Here's how the part is built. I have some questions about the finished solid (model axes, mm). Face numbers are marked on the shaded views. A direction names the side the tool comes from. Round coordinates to 2 decimals unless told otherwise and drop trailing zeros. Write each loop counter-clockwise with the first axis right and the second up, starting at its lowest first coordinate (ties: lowest second). Pieces come first, ordered by that corner, then holes. Notation, with made-up numbers: (67.5, 60.25) - (125.5, 60.25) arc R15 ccw to (125.5, 85.25) - close; hole circle Ø4 at (88.25, 69). An arc over 180 degrees is marked (long way). Write item = value, one per line. Start each with the question number.
Item 1: If we section it at B-B (y = 7): Please give me the cut outline in (x, z), and give its area (3 significant figures).
Item 2: Which directions (+Z, -Z, +X, -X, +Y, -Y) give clear straight access to the entire face, cutting with the end or side of a thin tool? Please do the marked faces 1, 2 and 3.
Item 3: If I drill on line 1 along X through (y, z) = (2, -6.75); line 2 along Z through (x, y) = (39, 7); line 3 along Y through (x, z) = (39.5, 0), over which ranges is the centre line in solid material (lowest first)? Write a range as [from, to].
Item 4: If we section it at C-C (x = 47): Please give me the cut outline in (y, z).
Item 5: For P1, Ø9.5, axis at x = 9.5, z = 10, coming from the +Y side; P2, Ø4, axis at y = 6.5, z = -2.5, coming from the +X side; P3, Ø2, axis at x = 47.5, y = 7.5, coming from the -Z side, each with a flat end and sliding along its axis, tell me the tip position at first contact or that it passes through.
Item 6: If we section it at D-D (z = 0): Please give me the cut outline in (x, y), and give its area (3 significant figures).
Item 7: Thinking about a two-plate mould opening in X: for the marked faces 4, 5, 6 and 7, which applies, pulls with the +X half, pulls with the -X half, needs draft (parallel to the pull), parting line crosses it, or undercut?
Item 8: If we section it at A-A (z = -6.75): Please give me the cut outline in (x, y).
```python
from build123d import *

# Parameters (mm, degrees)
EXTRUDE_2_DEPTH     = 4
SKETCH_7_W          = 100
SKETCH_7_H          = 16
EXTRUDE_3_DEPTH     = 6
SKETCH_8_R          = 5.25
CUT_EXTRUDE_3_DEPTH = 96
SKETCH_9_W          = 30
SKETCH_9_H          = 6
CUT_EXTRUDE_4_DEPTH = 94.680307429
SKETCH_10_R         = 1.8
CUT_EXTRUDE_5_DEPTH = 92.607859925
FILLET_3_R          = 15
CHAMFER_1_SIZE      = 1


with BuildPart() as part:
    # Эскиз6 → Бобышка-Вытянуть2 (new body)
    with BuildSketch(Plane(origin=(0, 0, 0), x_dir=(1, 0, 0), z_dir=(0, 1, 0))):
        Polygon((0, 16), (0, 8), (-10, 8), (-10, -8), (0, -8), (0, -16), (30, -16), (30, -8), (90, -8), (90, 8), (30, 8), (30, 16), align=None)
    extrude(amount=EXTRUDE_2_DEPTH)

    # Эскиз7 → Бобышка-Вытянуть3 (add)
    with BuildSketch(Plane(origin=(0, 4, 0), x_dir=(1, 0, 0), z_dir=(0, 1, 0))):
        with Locations((40, 0)):
            Rectangle(SKETCH_7_W, SKETCH_7_H)
    extrude(amount=EXTRUDE_3_DEPTH)

    # Эскиз8 → Вырез-Вытянуть3 (cut)
    with BuildSketch(Plane(origin=(90, 0, 0), x_dir=(0, 0, -1), z_dir=(1, 0, 0))):
        with Locations((0, 7)):
            Circle(SKETCH_8_R)
    extrude(amount=-CUT_EXTRUDE_3_DEPTH, mode=Mode.SUBTRACT)

    # Эскиз9 → Вырез-Вытянуть4 (cut, through all)
    with BuildSketch(Plane.XY.offset(8)):
        with Locations((15, 7)):
            Rectangle(SKETCH_9_W, SKETCH_9_H)
    extrude(amount=-CUT_EXTRUDE_4_DEPTH, mode=Mode.SUBTRACT)

    # Эскиз10 → Вырез-Вытянуть5 (cut, through all)
    with BuildSketch(Plane(origin=(0, 4, 0), x_dir=(1, 0, 0), z_dir=(0, 1, 0))):
        with Locations(Location((15, -13.5, 0), (0, 0, 270))):
            Circle(SKETCH_10_R)
        with Locations(Location((3.308657049, 6.75, 0), (0, 0, 270))):
            Circle(SKETCH_10_R)
        with Locations(Location((26.691342951, 6.75, 0), (0, 0, 270))):
            Circle(SKETCH_10_R)
    extrude(amount=-CUT_EXTRUDE_5_DEPTH, mode=Mode.SUBTRACT)

    # Скругление3
    # the kernel refuses this fillet: 15 mm, written as the material it takes off along each edge
    with BuildSketch(Plane(origin=(30, -33.166247904, -16), x_dir=(-1, 0, 0), z_dir=(0, 1, 0))) as fillet_3_piece_1:
        with BuildLine():
            CenterArc((13.266499161, 15), FILLET_3_R, 207.818139285, 62.181860715)
            Line((0, 8), (-0.265329983, 7.86))
            ThreePointArc((-0.265329983, 7.86), (-0.3, 4), (-0.3, 0))
            Line((-0.3, 0), (0, -0.3))
            Line((0, -0.3), (13.266499161, -0.3))
            Line((13.266499161, -0.3), (13.266499161, 0))
        make_face()
    extrude(amount=70.332495807, mode=Mode.SUBTRACT)
    with BuildSketch(Plane(origin=(0, -33.166247904, -16), x_dir=(0, 0, 1), z_dir=(0, 1, 0))) as fillet_3_piece_2:
        with BuildLine():
            CenterArc((15, 13.266499161), FILLET_3_R, 180, 62.181860715)
            Line((0, 13.266499161), (-0.3, 13.266499161))
            Line((-0.3, 13.266499161), (-0.3, 0))
            Line((-0.3, 0), (0, -0.3))
            ThreePointArc((0, -0.3), (4, -0.3), (7.86, -0.265329983))
            Line((7.86, -0.265329983), (8, 0))
        make_face()
    extrude(amount=70.332495807, mode=Mode.SUBTRACT)
    with BuildSketch(Plane(origin=(30, -33.166247904, 16), x_dir=(-1, 0, 0), z_dir=(0, 1, 0))) as fillet_3_piece_3:
        with BuildLine():
            CenterArc((13.266499161, -15), FILLET_3_R, 90, 62.181860715)
            Line((0, -8), (-0.265329983, -7.86))
            ThreePointArc((-0.265329983, -7.86), (-0.3, -4), (-0.3, 0))
            Line((-0.3, 0), (0, 0.3))
            Line((0, 0.3), (13.266499161, 0.3))
            Line((13.266499161, 0.3), (13.266499161, 0))
        make_face()
    extrude(amount=70.332495807, mode=Mode.SUBTRACT)
    with BuildSketch(Plane(origin=(0, -33.166247904, 16), x_dir=(0, 0, -1), z_dir=(0, 1, 0))) as fillet_3_piece_4:
        with BuildLine():
            CenterArc((15, -13.266499161), FILLET_3_R, 117.818139285, 62.181860715)
            Line((0, -13.266499161), (-0.3, -13.266499161))
            Line((-0.3, -13.266499161), (-0.3, 0))
            Line((-0.3, 0), (0, 0.3))
            ThreePointArc((0, 0.3), (4, 0.3), (7.86, 0.265329983))
            Line((7.86, 0.265329983), (8, 0))
        make_face()
    extrude(amount=70.332495807, mode=Mode.SUBTRACT)

    # Фаска1
    # the kernel refuses this chamfer: 1 mm, written as the material it takes off along each edge
    with BuildSketch(Plane(origin=(3.308657049, 4, -6.75), x_dir=(0, 0, 1), z_dir=(-1, 0, 0))) as chamfer_1_piece_1:
        Polygon((1.8, -CHAMFER_1_SIZE), (1.8 + CHAMFER_1_SIZE, 0), (1.8, 0), align=None)
    revolve(axis=Axis((3.308657049, 4, -6.75), (0, 1, 0)), mode=Mode.SUBTRACT)
    with BuildSketch(Plane(origin=(26.691342951, 4, -6.75), x_dir=(0, 0, 1), z_dir=(-1, 0, 0))) as chamfer_1_piece_2:
        Polygon((1.8, -CHAMFER_1_SIZE), (1.8 + CHAMFER_1_SIZE, 0), (1.8, 0), align=None)
    revolve(axis=Axis((26.691342951, 4, -6.75), (0, 1, 0)), mode=Mode.SUBTRACT)
    with BuildSketch(Plane(origin=(15, 4, 13.5), x_dir=(0, 0, 1), z_dir=(-1, 0, 0))) as chamfer_1_piece_3:
        Polygon((1.8, -CHAMFER_1_SIZE), (1.8 + CHAMFER_1_SIZE, 0), (1.8, 0), align=None)
    revolve(axis=Axis((15, 4, 13.5), (0, 1, 0)), mode=Mode.SUBTRACT)


solid = part.part
```
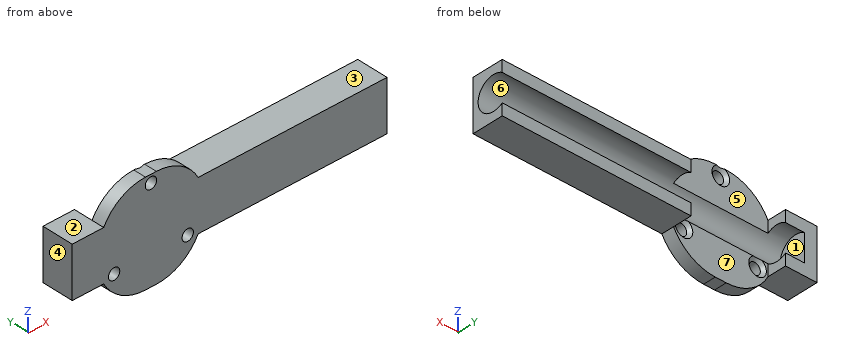
Reply:
q1.outline = (-10, -8) - (0, -8) - (0, -5.25) - (-6, -5.25) - (-6, 5.25) - (0, 5.25) - (0, 8) - (-10, 8) - close; (30, -8) - (90, -8) - (90, -5.25) - (30, -5.25) - close; (30, 5.25) - (90, 5.25) - (90, 8) - (30, 8) - close
q1.area = 427 mm2
q2.face_1 = +X
q2.face_2 = +Z, -X, +Y, -Y
q2.face_3 = +Z, +X, +Y, -Y
q3.line_1 = [-10, 1.51], [5.11, 24.89], [28.49, 90]
q3.line_2 = [-8, -5.25], [5.25, 8]
q3.line_3 = [0, 1.75]
q4.outline = (0, -8) - (10, -8) - (10, -4.31) arc R5.25 cw (long way) to (10, 4.31) - (10, 8) - (0, 8) - close
q5.P1 = 4
q5.P2 = -6
q5.P3 = -8
q6.outline = (-10, 0) - (90, 0) - (90, 1.75) - (-6, 1.75) - (-6, 10) - (-10, 10) - close
q6.area = 208 mm2
q7.face_4 = pulls with the -X half
q7.face_5 = undercut
q7.face_6 = needs draft
q7.face_7 = undercut
q8.outline = (-10, 0) - (1.51, 0) - (1.51, 3) - (0.51, 4) - (0, 4) - (0, 10) - (-10, 10) - close; (5.11, 0) - (24.89, 0) - (24.89, 3) - (23.89, 4) - (6.11, 4) - (5.11, 3) - close; (28.49, 0) - (90, 0) - (90, 10) - (30, 10) - (30, 4) - (29.49, 4) - (28.49, 3) - close
